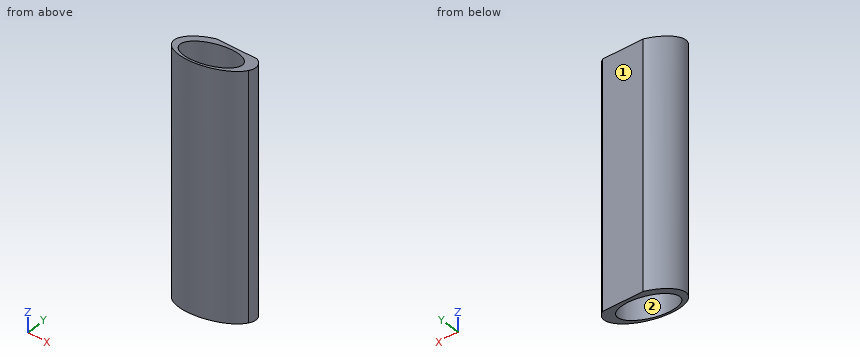
from build123d import *

# Parameters (mm, degrees)
F0_R          = 9.5
F1_DEPTH      = 100
F3_DEPTH      = 25
F3_DEPTH_BACK = 25


with BuildPart() as f1:
    # F0 (on Top) → F1 (new body)
    with BuildSketch(Plane.XY):
        with BuildLine():
            ThreePointArc((-7.5, 10), (-5.59017, -11.18034), (12.5, 0))
            ThreePointArc((12.5, 0), (11.18034, 5.59017), (7.5, 10))
            Line((7.5, 10), (-7.5, 10))
        make_face()
        with Locations((0, -1.666667)):
            Circle(F0_R, mode=Mode.SUBTRACT)
    extrude(amount=F1_DEPTH)


with BuildPart() as f3:
    # F2 (on Right) → F3 (new body, two sides)
    with BuildSketch(Plane.YZ) as f3_sk:
        Polygon((10, 100), (-12.5, 100), (10, 90.680195), align=None)
        Polygon((-12.5, 9.319805), (-12.5, 0), (10, 0), align=None)
    extrude(amount=F3_DEPTH)
    extrude(f3_sk.sketch, amount=-F3_DEPTH_BACK)


with BuildPart() as f1_1:
    add(f1.part)

    # F4: cut F3
    add(f3.part, mode=Mode.SUBTRACT)


solid = f1_1.part
Work out the finished part from the listing and answer in its coordinate system (mm). Face numbers are marked on the shaded views. Give positions to 0.01 mm unless a question says otherwise; leave off trailing zeros. Loops run counter-clockwise (first coordinate to the right, second up) from the corner with the lowest first, then second, coordinate; pieces in that order, holes last. Notation, with made-up numbers: (39, 79) -> (66, 79) arc R18 cw to (66, 112) -> close; hole circle Ø9 at (31.5, 13.5). An arc over 180 degrees is marked (long way). Use a Markdown table: item, result. Add a question column.
1) The part is cut by section A-A, the plane y = -8.25. Determine the outline of the cut face in (x, z), plus the area to 3 significant figures.
2) The part is cut by section B-B, the plane x = 1. Determine the outline of the cut face in (y, z), plus the area to 3 significant figures.
3) Consider line 1 along Y through (x, z) = (0, 29); line 2 along Y through (x, z) = (-5.5, 36.5); line 3 along X through (y, z) = (-4.75, 57). Determine where each line is inside the solid, lowest interval first.
4) Each of these flat-tipped pins is pushed along its axis until it touches: P1, Ø2, axis at y = 5.5, z = 79.5, coming from the +X side; P2, Ø5, axis at y = 6.5, z = 49.5, coming from the -X side; P3, Ø1, axis at x = -8, z = 66.5, coming from the -Y side; P4, Ø8, axis at x = -0.5, y = 1, coming from the -Z side. Where does it stop, or does it pass through?
5) For a pull along Y with two mould halves and no side action, classify the marked faces 1 and 2 as +Y half, -Y half, draft (parallel to the pull), parting line (faces both ways), or undercut.
6) The part is cut by section C-C, the plane z = 47. Determine the outline of the cut face in (x, y), plus the area to 3 significant figures.
Reported:
| question | item | result |
|---|---|---|
| 1 | outline | (-9.39, 7.56) -> (-6.85, 7.56) -> (-6.85, 98.24) -> (-9.39, 98.24) -> close; (6.85, 7.56) -> (9.39, 7.56) -> (9.39, 98.24) -> (6.85, 98.24) -> close |
| 1 | area | 461 mm^2 |
| 2 | outline | (-12.46, 9.3) -> (-11.11, 8.75) -> (-11.11, 99.43) -> (-12.46, 99.98) -> close; (7.78, 0.92) -> (10, 0) -> (10, 90.68) -> (7.78, 91.6) -> close |
| 2 | area | 323 mm^2 |
| 3 | line 1 | y = -12.5 to -11.17, 7.83 to 10 |
| 3 | line 2 | y = -11.22 to -9.41, 6.08 to 10 |
| 3 | line 3 | x = -11.56 to -8.99, 8.99 to 11.56 |
| 4 | P1 | stops at x = 11.66 |
| 4 | P2 | stops at x = -11.84 |
| 4 | P3 | stops at y = -10 |
| 4 | P4 | passes through |
| 5 | face 1 | +Y half |
| 5 | face 2 | undercut |
| 6 | outline | (-7.5, 10) arc R12.5 ccw (long way) to (12.5, 0) arc R12.5 ccw to (7.5, 10) -> close; hole circle Ø19 at (0, -1.67) |
| 6 | area | 182 mm^2 |
